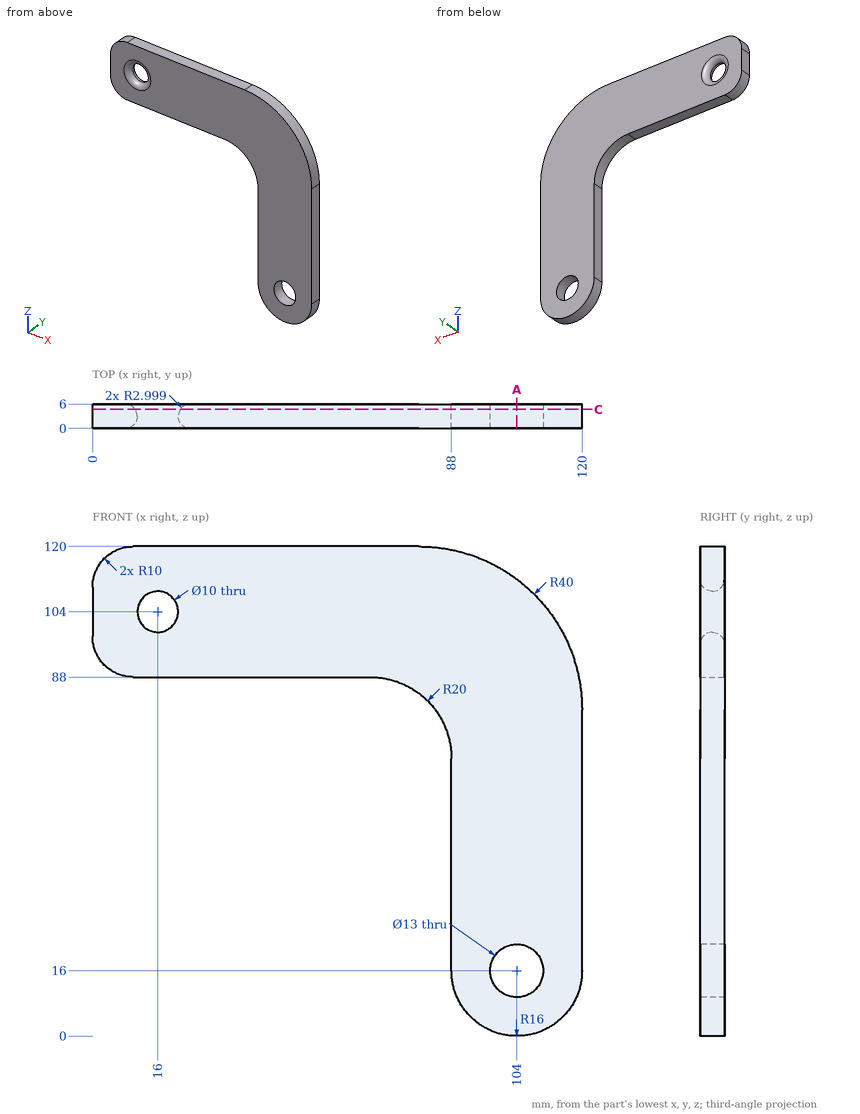
Here's the drawing with two shaded views (mm, measured from the low corner). I have some questions. Round coordinates to 2 decimals unless told otherwise and drop trailing zeros. Write each loop counter-clockwise with the first axis right and the second up, starting at its lowest first coordinate (ties: lowest second). Pieces come first, ordered by that corner, then holes.
(1) For pin 1 (13 mm diameter, centred on x = 16, z = 104, fed in from -Y); pin 2 (3 mm diameter, centred on y = 4.5, z = 45, fed in from -X); pin 3 (3 mm diameter, centred on x = 30, y = 2, fed in from -Z), each with a flat end and sliding along its axis, tell me the tip position at first contact or that it passes through.
Findings below:
pin 1: stops at y = 0.4
pin 2: stops at x = 88
pin 3: stops at z = 88
(2) If I drill on probe 1 along Z at (x, y) = (104, 3.55); probe 2 along Z at (x, y) = (16, 3.05); probe 3 along X at (y, z) = (3.8, 34), over which ranges is the centre line in solid material (lowest first)?
Findings below:
probe 1: z = 0 to 9.5, 22.5 to 112
probe 2: z = 88 to 99, 109 to 120
probe 3: x = 88 to 120
(3) Suppose I cut it at C-C on y = 4.7. Write out the boundary of the cut face in (x, z) (1 decimal).
Findings below:
outline: (0, 98) arc R10 ccw to (10, 88) - (68, 88) arc R20 cw to (88, 68) - (88, 16) arc R16 ccw to (120, 16) - (120, 80) arc R40 ccw to (80, 120) - (10, 120) arc R10 ccw to (0, 110) - close; hole circle Ø11.1 at (16, 104); hole circle Ø13 at (104, 16)
(4) Suppose I cut it at A-A on x = 104. Write out the boundary of the cut face in (y, z), and give its area (3 significant figures).
Findings below:
outline: (0, 0) - (6, 0) - (6, 9.5) - (0, 9.5) - close; (0, 22.5) - (6, 22.5) - (6, 112) - (0, 112) - close
area: 594 mm2
